from build123d import *

# Parameters (mm, degrees)
SKETCH1_R               = 1.6
BOSS_EXTRUDE1_DEPTH     = 4
CUT_EXTRUDE1_DEPTH      = 29.640006983
CUT_EXTRUDE1_DEPTH_BACK = 2


with BuildPart() as part:
    # Sketch1 → Boss-Extrude1 (new body)
    with BuildSketch(Plane(origin=(0, 0, 0), x_dir=(1, 0, 0), z_dir=(0, 1, 0))):
        Polygon((0, -22), (-4.5, -22), (-4.5, 28), (4.5, 28), (4.5, -22), align=None)
        with Locations(Location((0, -16, 0), (0, 0, 270))):
            Circle(SKETCH1_R, mode=Mode.SUBTRACT)
        with Locations(Location((0, 0, 0), (0, 0, 270))):
            Circle(SKETCH1_R, mode=Mode.SUBTRACT)
    extrude(amount=BOSS_EXTRUDE1_DEPTH)

    # Sketch2 → Cut-Extrude1 (cut, two sides: drawn at the far end of the back side and taken through both)
    with BuildSketch(Plane(origin=(0, 4, 0), x_dir=(1, 0, 0), z_dir=(0, 1, 0)).offset(-CUT_EXTRUDE1_DEPTH_BACK)):
        Polygon((-1, 138.603180864), (-1, 28), (-1, 8), (1, 8), (1, 28), (1, 138.603180864), (1, 359.809542593), (-1, 359.809542593), align=None)
    extrude(amount=CUT_EXTRUDE1_DEPTH + CUT_EXTRUDE1_DEPTH_BACK, mode=Mode.SUBTRACT)


solid = part.part
For this review, take the finished solid that the model builds, in its own axes (mm). A direction names the side the tool comes from. Give positions to 0.01 mm unless a question says otherwise; leave off trailing zeros. Order: outer loops, then holes, each group sorted by start corner. A loop starts at its lowest first (then second) coordinate and runs counter-clockwise, first axis right, second up. Notation, with made-up numbers: M -1,-16.75 L 21,-16.75 A11 ccw 21,-11.75 Z; hole C 29,23 d10. An arc over 180 degrees is marked long. Answer in a Markdown table with one row per item. Add a question column.
(1) Consider section A-A on z = 16. State the section outline as (x, y) points.
(2) Wall thickness on probe 1 along X at (y, z) = (2.8, -21); probe 2 along Z at (x, y) = (-0.75, 0.2); probe 3 along Z at (x, y) = (-1.25, 0.7): over which ranges is each line inside the solid? List them lowest first. Write a range as [from, to].
(3) Consider section B-B on z = -10. State the section outline as (x, y) points, and give its area (3 significant figures).
(4) For faces 4 (the face through (-4.5, 2, -3)), 5 (the face through (1, 3, -18)), list the 3-axis set-ups (+Z, -Z, +X, -X, +Y, -Y) from which the entire face can be reached by the end or side of a thin tool; tool diameter is ignored.
(5) Mouldability with a two-part tool opening along X and no side actions: class faces 1 (the face through (0, 3, -8)), 2 (the face through (-0.1, 1.5, -28)), 3 (the face through (4.5, 2, -3)) as +X half, -X half, draft (parallel to the pull), parting line (faces both ways), or undercut.
(6) For pin 1 (1 mm diameter, centred on x = 0, z = -16.5, fed in from +Y), flat-tipped, find the tip position at first contact; note if it passes through.
Evaluation:
| question | item | result |
|---|---|---|
| 1 | outline | M -4.5,0 L -1.6,0 L -1.6,4 L -4.5,4 Z; M 1.6,0 L 4.5,0 L 4.5,4 L 1.6,4 Z |
| 2 | probe 1 | x = [-4.5, -1], [1, 4.5] |
| 2 | probe 2 | z = [-28, -1.41], [1.41, 14.59], [17.41, 22] |
| 2 | probe 3 | z = [-28, -1], [1, 15], [17, 22] |
| 3 | outline | M -4.5,0 L 4.5,0 L 4.5,4 L 1,4 L 1,2 L -1,2 L -1,4 L -4.5,4 Z |
| 3 | area | 32.0 mm^2 |
| 4 | face 4 | +Z, -Z, -X, +Y, -Y |
| 4 | face 5 | -Z, +Y |
| 5 | face 1 | undercut |
| 5 | face 2 | draft |
| 5 | face 3 | +X half |
| 6 | pin 1 | stops at y = 2 |
